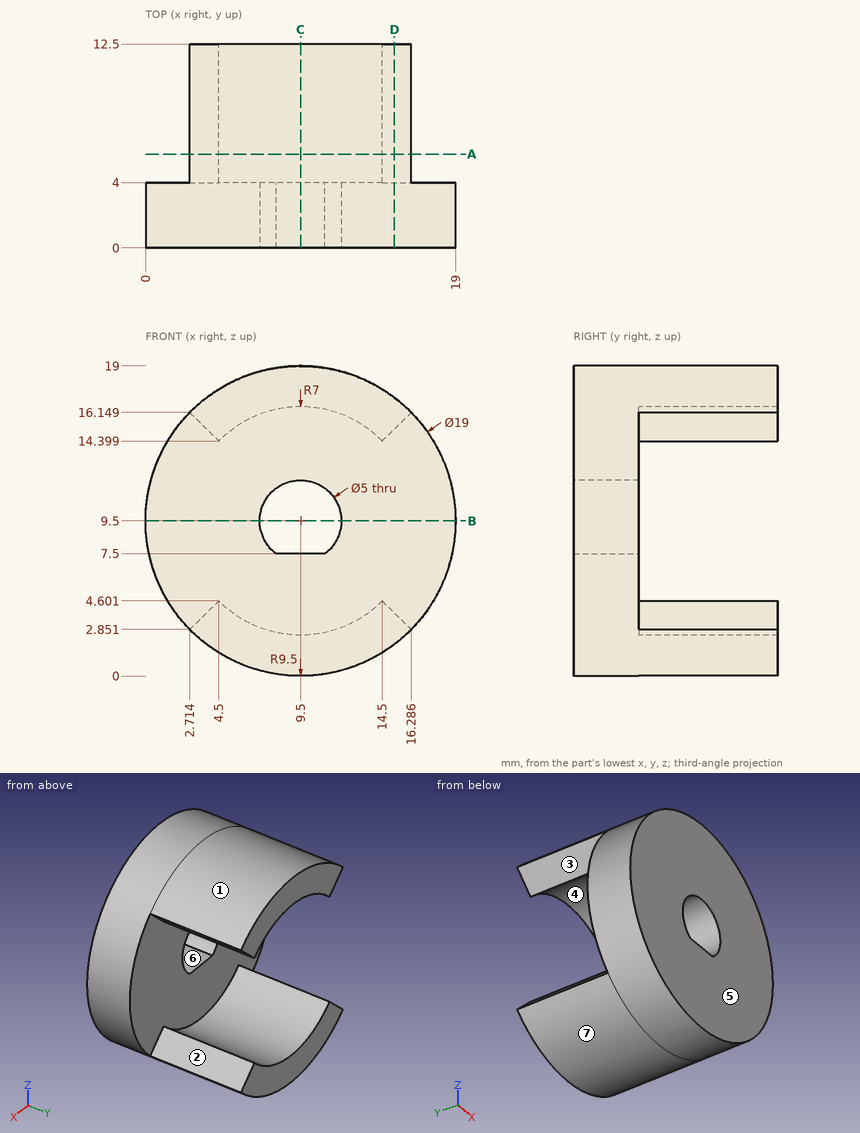
Here's the drawing with two shaded views (mm, measured from the low corner). I have some questions. A direction names the side the tool comes from. Coordinates: 2 decimals unless noted, no trailing zeros. Order: outer loops, then holes, each group sorted by start corner. A loop starts at its lowest first (then second) coordinate and runs counter-clockwise, first axis right, second up. Notation, with made-up numbers: M 46,8 L 80,8 A17 cw 80,24 Z; hole C 11,37.25 d10. An arc over 180 degrees is marked long. Write item = value, one per line.
(1) For the marked faces 1, 2, 3 and 4, which set-ups out of +Z, -Z, +X, -X, +Y, -Y let a thin tool reach every point of the face, with its end or its side?
Results are:
face_1 = +Z, +Y, -Y
face_2 = +X, +Y
face_3 = -X, +Y
face_4 = +Y
(2) Suppose I cut it at D-D on x = 15.25. Please give me the cut outline in (y, z).
Results are:
outline = M 0,1.94 L 12.5,1.94 L 12.5,3.87 L 4,3.87 L 4,15.13 L 12.5,15.13 L 12.5,17.06 L 0,17.06 Z
(3) If we mould it in two halves opening along X, with no side actions, what happens to the marked faces 5, 6 and 7? For each: pulls with the +X half, pulls with the -X half, needs draft (parallel to the pull), parting line crosses it, or undercut.
Results are:
face_5 = needs draft
face_6 = undercut
face_7 = parting line crosses it
(4) I need wall thicknesses on line 1 along X through (y, z) = (1, 9.5); line 2 along Z through (x, y) = (9.5, 2.5); line 3 along Y through (x, z) = (16.75, 7). Which ranges of each line are inside material? Lowest first, please. Write a range as [from, to].
Results are:
line_1 = [0, 7], [12, 19]
line_2 = [0, 7.5], [12, 19]
line_3 = [0, 4]
(5) Suppose I cut it at C-C on x = 9.5. Please give me the cut outline in (y, z).
Results are:
outline = M 0,0 L 12.5,0 L 12.5,2.5 L 4,2.5 L 4,7.5 L 0,7.5 Z; M 0,12 L 4,12 L 4,16.5 L 12.5,16.5 L 12.5,19 L 0,19 Z
(6) For pin 1 Ø4 at (x, z) = (6.5, 10) entering from +Y; pin 2 Ø2 at (y, z) = (3.5, 7.5) entering from -X; pin 3 Ø6 at (x, y) = (2.5, 9) entering from -Z, each with a flat end and sliding along its axis, tell me the tip position at first contact or that it passes through.
Results are:
pin_1 = 4
pin_2 = 0.05
pin_3 = 0.88
(7) Suppose I cut it at B-B on z = 9.5. Please give me the cut outline in (x, y), plus the area to 3 significant figures.
Results are:
outline = M 0,0 L 7,0 L 7,4 L 0,4 Z; M 12,0 L 19,0 L 19,4 L 12,4 Z
area = 56.0 mm2
(8) Suppose I cut it at A-A on y = 5.75. Please give me the cut outline in (x, z) (1 decimal).
Results are:
outline = M 2.7,2.9 A9.5 ccw 16.3,2.9 L 14.5,4.6 A7 cw 4.5,4.6 Z; M 2.7,16.1 L 4.5,14.4 A7 cw 14.5,14.4 L 16.3,16.1 A9.5 ccw Z
